Design review of the part shown in the three views and the two pictorial views. Dimensions are in mm from the part's minimum x, y and z. Round coordinates to 2 decimals unless told otherwise and drop trailing zeros. Order: outer loops, then holes, each group sorted by start corner. A loop starts at its lowest first (then second) coordinate and runs counter-clockwise, first axis right, second up.
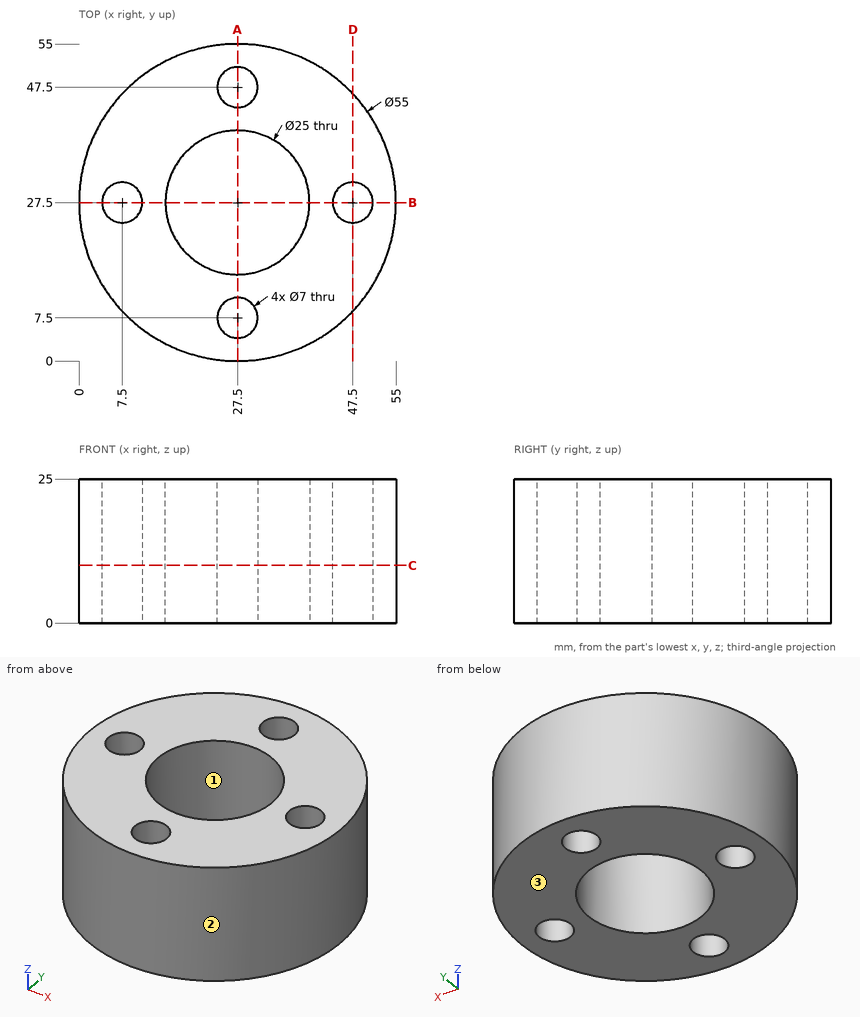
1) Take a section at D-D on x = 47.5. Give the boundary of the cut face in (y, z), plus the area to 3 significant figures.
Results:
outline: (8.63, 0) - (24, 0) - (24, 25) - (8.63, 25) - close; (31, 0) - (46.37, 0) - (46.37, 25) - (31, 25) - close
area: 769 mm2
2) The part is to be moulded in two halves that separate along Y. For the marked faces 1, 2 and 3, say which applies: released by +Y, released by -Y, zero draft, split by the parting line, or undercut.
Results:
face 1: undercut
face 2: split by the parting line
face 3: zero draft
3) Take a section at C-C on z = 10. Give the boundary of the cut face in (x, y), plus the area to 3 significant figures.
Results:
outline: circle Ø55 at (27.5, 27.5); hole circle Ø7 at (7.5, 27.5); hole circle Ø25 at (27.5, 27.5); hole circle Ø7 at (27.5, 7.5); hole circle Ø7 at (27.5, 47.5); hole circle Ø7 at (47.5, 27.5)
area: 1,730 mm2
4) To check wall thickness, follow line 1 along Y through (x, z) = (27.5, 18); line 2 along X through (y, z) = (26, 5.5); line 3 along X through (y, z) = (45, 8.75). State the ranges of each line that lie inside material, in increasing order.
Results:
line 1: y = 0 to 4, 11 to 15, 40 to 44, 51 to 55
line 2: x = 0.04 to 4.34, 10.66 to 15.09, 39.91 to 44.34, 50.66 to 54.96
line 3: x = 6.29 to 25.05, 29.95 to 48.71
5) Take a section at A-A on x = 27.5. Give the boundary of the cut face in (y, z), plus the area to 3 significant figures.
Results:
outline: (0, 0) - (4, 0) - (4, 25) - (0, 25) - close; (11, 0) - (15, 0) - (15, 25) - (11, 25) - close; (40, 0) - (44, 0) - (44, 25) - (40, 25) - close; (51, 0) - (55, 0) - (55, 25) - (51, 25) - close
area: 400 mm2
6) Clearance check with flat-ended pins moving along their axes: P1, Ø12, axis at y = 48, z = 19.5, coming from the +X side; P2, Ø15, axis at x = 27.5, y = 27.5, coming from the -Z side; P3, Ø12, axis at x = 21, z = 10, coming from the +Y side; P4, Ø1.5, axis at x = 36, z = 15, coming from the +Y side. State where each tip first meets the part, or that it passes through.
Results:
P1: stops at x = 50.87
P2: passes through
P3: stops at y = 55
P4: stops at y = 53.89
